```python
from build123d import *

# Parameters (mm, degrees)
DOME1_FACE_RADIUS = 3.302
DOME1_HEIGHT      = 2.54
SEEDCUT_DEPTH     = 21.698272826
CIRPATTERN1_COUNT = 8


# Read off the part's stored shape, not the designer's step: Cut-Revolve-Thin4
with BuildPart() as part:
    # Sketch1 → Revolve1 (revolve)
    with BuildSketch(Plane(origin=(0, 0, 0), x_dir=(0, 0, -1), z_dir=(1, 0, 0)), mode=Mode.PRIVATE) as revolve1_sk:
        Polygon((-2.54, 0), (-2.54, 7.493), (0, 7.493), (0, 5.08), (12.7, 5.08), (12.7, 0), align=None)
    revolve(revolve1_sk.sketch.rotate(Axis((0, 0, 12.072762836), (0, 0, -1)), 90), axis=Axis((0, 0, 12.072762836), (0, 0, -1)))

    # Sketch3 → Revolve2 (revolve)
    with BuildSketch(Plane(origin=(0, 0, 0), x_dir=(0, 0, -1), z_dir=(1, 0, 0))):
        with BuildLine():
            Line((-12.887595566, 0), (-2.54, 0))
            Line((-2.54, 0), (-2.54, 5.984091271))
            add(Edge.make_bspline(
                [(-2.54, 5.984091271), (-9.10319215, 5.770912184), (-12.887595566, 0)],
                knots=[0, 0, 0, 1, 1, 1], degree=2))
        make_face()
    revolve(axis=Axis((0, 0, 12.072762836), (0, 0, 1)))

    # Cut-Revolve-Thin4 outline → Cut-Revolve-Thin4 (revolve, cut)
    with BuildSketch(Plane.XZ):
        Polygon((3.302, -10.922), (3.302, -12.7), (5.08, -12.7), (5.08, -6.35), align=None)
    revolve(axis=Axis((0, 0, 0), (0, 0, 1)), mode=Mode.SUBTRACT)

    # Dome1: a dome of height H over a round flat face of radius A is a cap of a sphere of radius (A * A + H * H) / (2 * H)
    dome1_r = (DOME1_FACE_RADIUS * DOME1_FACE_RADIUS + DOME1_HEIGHT * DOME1_HEIGHT) / (2 * DOME1_HEIGHT)
    dome1_base = Plane((0, 0, -12.7), z_dir=(0, 0, -1))
    with Locations(dome1_base.offset(DOME1_HEIGHT - dome1_r)):
        dome1_ball = Sphere(dome1_r, mode=Mode.PRIVATE)
    add(split(dome1_ball, bisect_by=dome1_base, keep=Keep.TOP, mode=Mode.PRIVATE))

    # Sketch6 → SeedCut (cut, through all)
    with BuildSketch(Plane.XY.offset(2.54)):
        with BuildLine():
            Line((0.217011402, 6.735050359), (0.959619925, 7.431297235))
            ThreePointArc((0.959619925, 7.431297235), (0.241308217, 7.489113388), (-0.479235475, 7.477658882))
            Line((-0.479235475, 7.477658882), (0.217011402, 6.735050359))
        make_face()
    seedcut = extrude(amount=-SEEDCUT_DEPTH, mode=Mode.SUBTRACT)

    # CirPattern1: SeedCut ×8 about axis
    cirpattern1_axis = Axis((0, 0, 0), (0, 0, 1))
    for i in range(1, CIRPATTERN1_COUNT):
        add(seedcut.rotate(cirpattern1_axis, i * 360 / CIRPATTERN1_COUNT), mode=Mode.SUBTRACT)


solid = part.part
```
The model under review builds one solid part; all positions refer to its coordinate system, in mm. A direction names the side the tool comes from. Round coordinates to 2 decimals unless told otherwise and drop trailing zeros. Write each loop counter-clockwise with the first axis right and the second up, starting at its lowest first coordinate (ties: lowest second). Pieces come first, ordered by that corner, then holes. Notation, with made-up numbers: (21.25, 44.25) - (49.25, 44.25) arc R16 cw to (49.25, 60.25) - close; hole circle Ø3 at (-22.5, -9.75). An arc over 180 degrees is marked (long way). One line per question, with ' | ' between items.
Item 1: To check wall thickness, follow probe 1 along X at (y, z) = (1, 1.75); probe 2 along Y at (x, z) = (-1.5, -8.75); probe 3 along X at (y, z) = (-3.5, 8.75). State the ranges of each line that lie inside material, in increasing order.
Resolved:
probe 1: x = -7.43 to 7.43 | probe 2: y = -3.87 to 3.87 | probe 3: x = -2.28 to 2.28
Item 2: Add section A-A, the plane z = 0.75. Give the boundary of the cut face in (x, y).
Resolved:
outline: (-7.48, -0.48) arc R7.49 ccw to (-5.93, -4.58) - (-4.92, -4.61) - (-4.95, -5.63) arc R7.49 ccw to (-0.96, -7.43) - (-0.22, -6.74) - (0.48, -7.48) arc R7.49 ccw to (4.58, -5.93) - (4.61, -4.92) - (5.63, -4.95) arc R7.49 ccw to (7.43, -0.96) - (6.74, -0.22) - (7.48, 0.48) arc R7.49 ccw to (5.93, 4.58) - (4.92, 4.61) - (4.95, 5.63) arc R7.49 ccw to (0.96, 7.43) - (0.22, 6.74) - (-0.48, 7.48) arc R7.49 ccw to (-4.58, 5.93) - (-4.61, 4.92) - (-5.63, 4.95) arc R7.49 ccw to (-7.43, 0.96) - (-6.74, 0.22) - close
Item 3: For faces 1 (the face through (-6.84, 3.06, 1.25)), 2 (the face through (3.05, -1.26, -11.82)), 3 (the face through (6, 2, 2.54)), list the 3-axis set-ups (+Z, -Z, +X, -X, +Y, -Y) from which the entire face can be reached by the end or side of a thin tool; tool diameter is ignored.
Resolved:
face 1: +Z, -Z, -X, +Y | face 2: -Z | face 3: +Z
Item 4: Add section B-B, the plane z = -13.25. Give the boundary of the cut face in (x, y).
Resolved:
outline: circle Ø6.21 at (0, 0)
Item 5: For P1, Ø1.5, axis at y = -1, z = 6, coming from the -X side; P2, Ø2, axis at y = 1, z = -6, coming from the +X side; P3, Ø1, axis at x = 0.5, y = 2.5, coming from the +Z side, all flat-tipped, find the tip position at first contact; note any pin that passes through.
Resolved:
P1: stops at x = -5.57 | P2: stops at x = 5.08 | P3: stops at z = 11.3
